Drawing for the job (mm, zero at the part's lowest x, y, z). Round coordinates to 2 decimals unless told otherwise and drop trailing zeros. Write each loop counter-clockwise with the first axis right and the second up, starting at its lowest first coordinate (ties: lowest second). Pieces come first, ordered by that corner, then holes.
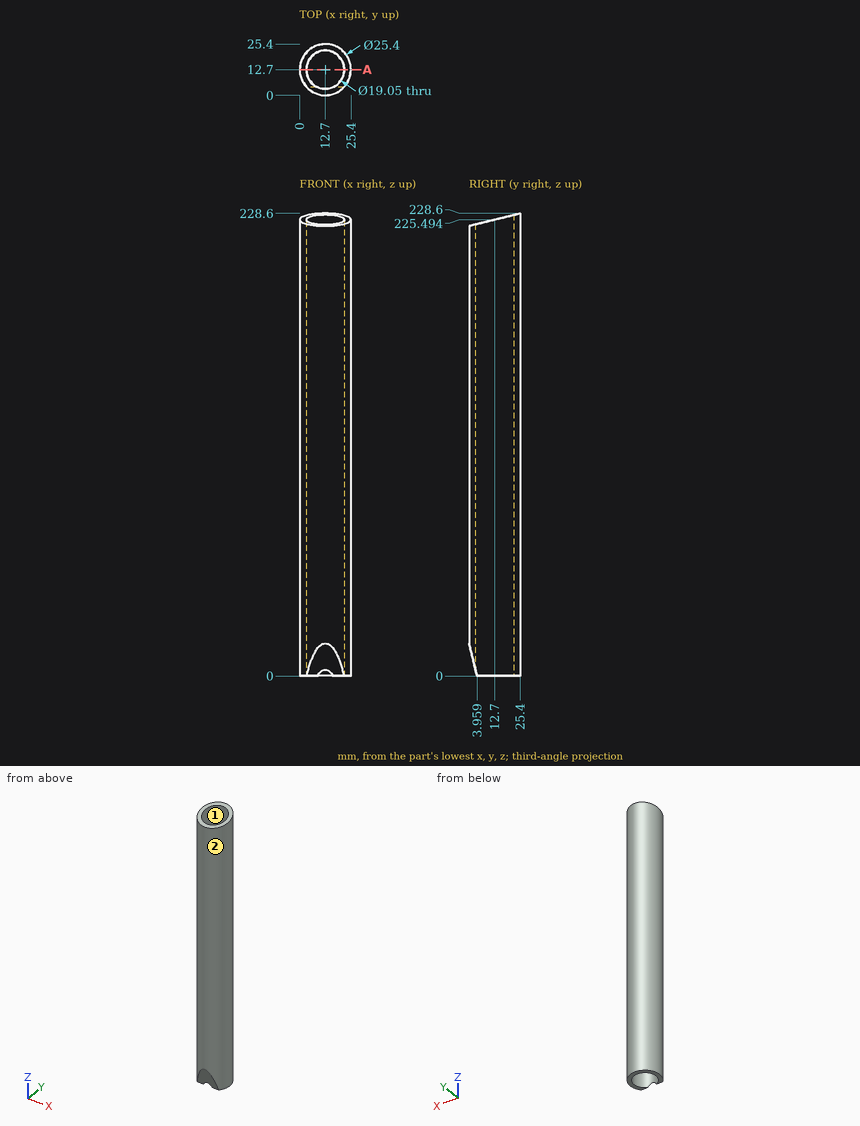
Q1. Drop flat-ended pins along their axis: P1, Ø3, axis at x = 19, y = 4, coming from the +Z side; P2, Ø1, axis at x = 11, z = 169, coming from the +Y side; P3, Ø1.5, axis at x = 4.5, y = 6, coming from the +Z side. Give the stop position or say it passes through.
Q2. Saw through at A-A, the plane y = 12.7. Write the cut outline in (x, z) (1 decimal), and give its area (3 significant figures).
Q3. Wall check: line 1 (Y direction, x = 12.7, z = 63.5) (1 decimal); line 2 (Y direction, x = 9, z = 51.5). Give the ranges that are in metal, low to high.
Q4. Two-plate mould, pull along Y, no slides. Class the marked faces 1 and 2: released by +Y, released by -Y, zero draft, split by the parting line, or undercut.
Computed:
1. P1: stops at z = 223.73
1. P2: stops at y = 25.34
1. P3: stops at z = 224.04
2. outline: (0, 0) - (3.2, 0) - (3.2, 225.5) - (0, 225.5) - close; (22.2, 0) - (25.4, 0) - (25.4, 225.5) - (22.2, 225.5) - close
2. area: 1,430 mm2
3. line 1: y = 0 to 3.2, 22.2 to 25.4
3. line 2: y = 0.55 to 3.92, 21.48 to 24.85
4. face 1: undercut
4. face 2: split by the parting line
